CAD build for the part. Positions are in the model's coordinates, mm. A direction names the side the tool comes from. Give positions to 0.01 mm unless a question says otherwise; leave off trailing zeros. Order: outer loops, then holes, each group sorted by start corner. A loop starts at its lowest first (then second) coordinate and runs counter-clockwise, first axis right, second up.
Item 1: Which spindle directions (+Z, -Z, +X, -X, +Y, -Y) get a long thin tool onto all of the face, cutting with end or side? Do faces 1 (the cylindrical face through (-18.462, -4.014, -8.708)), 2 (the flat face through (4.5, 22, -22)), 3 (the cylindrical face through (6.533, 11.832, 20.746)). Say none if no direction does.
Item 2: Flat gauge pins, fed straight in: P1, Ø8, axis at y = 0.5, z = -14, coming from the +X side; P2, Ø0.7, axis at y = 22.5, z = -22.5, coming from the +X side; P3, Ø1.1, axis at y = 23, z = -22.5, coming from the -X side. Where does each tip first touch, or does it go through?
Item 3: Band-saw the part on A-A on z = 0. Give the cut face in (x, y).
Item 4: Band-saw the part on B-B on x = 0. Give the cut face in (y, z), plus the area to 3 significant figures.
Item 5: Wall check: L1, parallel to X at y = -3.8, z = -9.25; L2, parallel to X at y = 9.5, z = 9.5; L3, parallel to X at y = -3.5, z = 18.5. Give the ranges that are in metal, low to high.
Item 6: Two-plate mould, pull along X, no slides. Class faces 4 (the cylindrical face through (13.58, -4.01, -8.71)), 5 (the flat face through (5.45, 24, 21.25)): released by +X, released by -X, zero draft, split by the parting line, or undercut.
Item 7: Band-saw the part on D-D on y = 3. Give the cut face in (x, z).
Item 8: Band-saw the part on C-C on z = -10. Give the cut face in (x, y).
```python
from build123d import *

# Parameters (mm, degrees)
SKETCH1_R               = 24
SKETCH1_R_2             = 21.75
BOSS_EXTRUDE1_DEPTH     = 24
BOSS_EXTRUDE2_START     = 5
SKETCH2_R               = 24
SKETCH2_R_2             = 15
BOSS_EXTRUDE2_DEPTH     = 5
SKETCH3_R               = 2.5
CUT_EXTRUDE1_DEPTH      = 2
SKETCH4_R               = 1.5
CUT_EXTRUDE2_DEPTH      = 44.370496884
CUT_EXTRUDE3_REACH      = 60.788
CUT_EXTRUDE3_END_RADIUS = 21.75
SKETCH5_W               = 9
SKETCH5_H               = 4


with BuildPart() as part:
    # Sketch1 → Boss-Extrude1 (new body)
    with BuildSketch(Plane(origin=(0, 0, 0), x_dir=(1, 0, 0), z_dir=(0, 1, 0))):
        with Locations(Location((0, 0, 0), (0, 0, 270))):
            Circle(SKETCH1_R)
        with Locations(Location((0, 0, 0), (0, 0, 270))):
            Circle(SKETCH1_R_2, mode=Mode.SUBTRACT)
    extrude(amount=BOSS_EXTRUDE1_DEPTH)

    # Sketch2 → Boss-Extrude2 (add)
    with BuildSketch(Plane.XZ.offset(BOSS_EXTRUDE2_START)):
        with Locations(Location((0, 0, 0), (0, 0, 270))):
            Circle(SKETCH2_R)
        with Locations(Location((0, 0, 0), (0, 0, 270))):
            Circle(SKETCH2_R_2, mode=Mode.SUBTRACT)
    extrude(amount=-BOSS_EXTRUDE2_DEPTH)

    # Sketch3 → Cut-Extrude1 (cut)
    with BuildSketch(Plane.XZ.offset(5)):
        with Locations(Location((0, 18.5, 0), (0, 0, 270))):
            Circle(SKETCH3_R)
        with Locations(Location((16.02146997, -9.25, 0), (0, 0, 270))):
            Circle(SKETCH3_R)
        with Locations(Location((-16.02146997, -9.25, 0), (0, 0, 270))):
            Circle(SKETCH3_R)
    extrude(amount=-CUT_EXTRUDE1_DEPTH, mode=Mode.SUBTRACT)

    # Sketch4 → Cut-Extrude2 (cut, through all)
    with BuildSketch(Plane.XZ.offset(3)):
        with Locations(Location((0, 18.5, 0), (0, 0, 270))):
            Circle(SKETCH4_R)
        with Locations(Location((16.02146997, -9.25, 0), (0, 0, 270))):
            Circle(SKETCH4_R)
        with Locations(Location((-16.02146997, -9.25, 0), (0, 0, 270))):
            Circle(SKETCH4_R)
    extrude(amount=-CUT_EXTRUDE2_DEPTH, mode=Mode.SUBTRACT)

    # Cut-Extrude3: up to this cylinder (the profile starts outside it)
    cut_extrude3_end = Plane(origin=(0, 22, 0), z_dir=(0, -1, 0)) * Cylinder(CUT_EXTRUDE3_END_RADIUS, 166.076, mode=Mode.PRIVATE)
    # Sketch5 → Cut-Extrude3 (cut, up to the surface)
    with BuildSketch(Plane(origin=(0, 0, -24), x_dir=(-1, 0, 0), z_dir=(0, 0, -1)), mode=Mode.PRIVATE) as cut_extrude3_sk1:
        with Locations((0, 22)):
            Rectangle(SKETCH5_W, SKETCH5_H)
    cut_extrude3_tool1 = extrude(cut_extrude3_sk1.sketch, amount=-CUT_EXTRUDE3_REACH, mode=Mode.PRIVATE) - cut_extrude3_end
    add(cut_extrude3_tool1.solids().sort_by_distance((0, 22, -24))[0], mode=Mode.SUBTRACT)


solid = part.part
```
The answers:
1. face 1: -Y
1. face 2: -Z, +Y
1. face 3: +Y
2. P1: stops at x = 21.82
2. P2: stops at x = 9.24
2. P3: stops at x = -9.71
3. outline: (-24, -5) - (-15, -5) - (-15, 0) - (-21.75, 0) - (-21.75, 24) - (-24, 24) - close; (15, -5) - (24, -5) - (24, 24) - (21.75, 24) - (21.75, 0) - (15, 0) - close
4. outline: (-5, -24) - (20, -24) - (20, -21.75) - (0, -21.75) - (0, -15) - (-5, -15) - close; (-5, 15) - (0, 15) - (0, 17) - (-3, 17) - (-3, 16) - (-5, 16) - close; (-5, 21) - (-3, 21) - (-3, 20) - (0, 20) - (0, 21.75) - (24, 21.75) - (24, 24) - (-5, 24) - close
4. area: 170 mm2
5. L1: x = -22.15 to -18.52, -13.52 to -11.81, 11.81 to 13.52, 18.52 to 22.15
5. L2: x = -22.04 to -19.57, 19.57 to 22.04
5. L3: x = -15.29 to -2.5, 2.5 to 15.29
6. face 4: undercut
6. face 5: zero draft
7. outline: circle Ø48 at (0, 0); hole circle Ø43.5 at (0, 0)
8. outline: (-21.82, -5) - (-18.41, -5) - (-18.41, -3) - (-17.32, -3) - (-17.32, 0) - (-19.31, 0) - (-19.31, 24) - (-21.82, 24) - close; (-14.72, -3) - (-13.64, -3) - (-13.64, -5) - (-11.18, -5) - (-11.18, 0) - (-14.72, 0) - close; (11.18, -5) - (13.64, -5) - (13.64, -3) - (14.72, -3) - (14.72, 0) - (11.18, 0) - close; (17.32, -3) - (18.41, -3) - (18.41, -5) - (21.82, -5) - (21.82, 24) - (19.31, 24) - (19.31, 0) - (17.32, 0) - close
